from build123d import *

# Parameters (mm, degrees)
SKETCH1_R           = 2
BOSS_EXTRUDE1_DEPTH = 2
CUT_EXTRUDE1_REACH  = 41.7
SKETCH2_R           = 6


with BuildPart() as part:
    # Sketch1 → Boss-Extrude1 (new body)
    with BuildSketch(Plane(origin=(0, 0, 0), x_dir=(1, 0, 0), z_dir=(0, 1, 0))):
        with BuildLine():
            Line((-6, 37), (6, 37))
            Line((6, 37), (6, 12.925265955))
            ThreePointArc((6, 12.925265955), (14.25, 0), (6, -12.925265955))
            Line((6, -12.925265955), (6, -37))
            Line((6, -37), (-6, -37))
            Line((-6, -37), (-6, -12.925265955))
            ThreePointArc((-6, -12.925265955), (-14.25, 0), (-6, 12.925265955))
            Line((-6, 12.925265955), (-6, 37))
        make_face()
        with Locations(Location((0, 32.5, 0), (0, 0, 270))):
            Circle(SKETCH1_R, mode=Mode.SUBTRACT)
        with Locations(Location((0, -32.5, 0), (0, 0, 90))):
            Circle(SKETCH1_R, mode=Mode.SUBTRACT)
    extrude(amount=BOSS_EXTRUDE1_DEPTH)

    # Sketch2 → Cut-Extrude1 (cut, up to next)
    with BuildSketch(Plane(origin=(0, 2, 0), x_dir=(1, 0, 0), z_dir=(0, 1, 0)), mode=Mode.PRIVATE) as cut_extrude1_sk1:
        with Locations(Location((0, 0, 0), (0, 0, 270))):
            Circle(SKETCH2_R)
    cut_extrude1_tool1 = extrude(cut_extrude1_sk1.sketch, amount=-CUT_EXTRUDE1_REACH, mode=Mode.PRIVATE) & part.part
    add(cut_extrude1_tool1.solids().sort_by_distance((0, 2, 0))[0], mode=Mode.SUBTRACT)


solid = part.part
Check sheet for the modelled part. Datum: model origin and axes. Units: mm. A direction names the side the tool comes from. Round coordinates to 2 decimals unless told otherwise and drop trailing zeros. Loops run counter-clockwise (first coordinate to the right, second up) from the corner with the lowest first, then second, coordinate; pieces in that order, holes last.
1. Sectioned sample at D-D on z = -15. Record the boundary of the cut face in (x, y), and give its area (3 significant figures).
2. Gauge pin test, flat ends, axial feed: pin 1 Ø3 at (x, z) = (0, -32.5) entering from -Y; pin 2 Ø6.5 at (x, z) = (0, 32.5) entering from -Y; pin 3 Ø0.6 at (y, z) = (1, 25) entering from +X; pin 4 Ø1 at (x, y) = (9.5, 1) entering from +Z. Record the tip position at first contact, or that the pin passes through.
3. Mould release check, pull along Z, two halves, no side actions. Record for faces 1 (the cylindrical face through (0.766, 0.986, 30.653)), 2 (the flat face through (7, 2, -1)), 3 (the flat face through (0, 1, -37)), 4 (the cylindrical face through (-14.25, 0.99, 0.23)): released by +Z, released by -Z, zero draft, split by the parting line, or undercut.
4. Sectioned sample at C-C on x = 4. Record the boundary of the cut face in (y, z).
5. Scan lines: probe 1 along Z at (x, y) = (0.75, 0.3); probe 2 along X at (y, z) = (1.35, -32.5); probe 3 along X at (y, z) = (0.2, 26). Record each from-to range of solid material in increasing order.
6. Sectioned sample at A-A on z = 32.5. Record the boundary of the cut face in (x, y).
7. Sectioned sample at B-B on y = 0.95. Record the boundary of the cut face in (x, z).
8. Set-up check for faces 5 (the flat face through (6, 1, -25)), 6 (the flat face through (6, 1, 25)), 7 (the flat face through (7, 0, -1)), 8 (the flat face through (-6, 1, 25)), 9 (the flat face through (-6, 1, -25)): record each of +Z, -Z, +X, -X, +Y, -Y from which the full face is reachable in a straight line by a thin tool's end or side.
Recorded:
1. outline: (-6, 0) - (6, 0) - (6, 2) - (-6, 2) - close
1. area: 24.0 mm2
2. pin 1: passes through
2. pin 2: stops at y = 0
2. pin 3: stops at x = 6
2. pin 4: stops at z = 11.05
3. face 1: undercut
3. face 2: zero draft
3. face 3: released by -Z
3. face 4: split by the parting line
4. outline: (0, -37) - (2, -37) - (2, -4.47) - (0, -4.47) - close; (0, 4.47) - (2, 4.47) - (2, 37) - (0, 37) - close
5. probe 1: z = -37 to -34.35, -30.65 to -5.95, 5.95 to 30.65, 34.35 to 37
5. probe 2: x = -6 to -2, 2 to 6
5. probe 3: x = -6 to 6
6. outline: (-6, 0) - (-2, 0) - (-2, 2) - (-6, 2) - close; (2, 0) - (6, 0) - (6, 2) - (2, 2) - close
7. outline: (-6, -37) - (6, -37) - (6, -12.93) arc R14.25 ccw to (6, 12.93) - (6, 37) - (-6, 37) - (-6, 12.93) arc R14.25 ccw to (-6, -12.93) - close; hole circle Ø12 at (0, 0); hole circle Ø4 at (0, -32.5); hole circle Ø4 at (0, 32.5)
8. face 5: -Z, +X, +Y, -Y
8. face 6: +Z, +X, +Y, -Y
8. face 7: +Z, -Z, +X, -X, -Y
8. face 8: +Z, -X, +Y, -Y
8. face 9: -Z, -X, +Y, -Y
